Check sheet for the modelled part. Datum: model origin and axes. Units: mm. A direction names the side the tool comes from. Coordinates: 2 decimals unless noted, no trailing zeros. Loops run counter-clockwise (first coordinate to the right, second up) from the corner with the lowest first, then second, coordinate; pieces in that order, holes last. Notation, with made-up numbers: (49, 45) -> (86, 45) arc R11 cw to (86, 50) -> close; hole circle Ø1 at (81, 21). An arc over 180 degrees is marked (long way). Use CSV: the item, a comma, the result in double quotes. Start each with the question number.
1. Set-up check for faces 4 (the face through (69.6, -59.9, 9.7)), 5 (the face through (3, -57.219, 21)), 6 (the face through (68.086, 44.779, 3.346)): record each of +Z, -Z, +X, -X, +Y, -Y from which the full face is reachable in a straight line by a thin tool's end or side.
2. Sectioned sample at A-A, the plane z = 3.75. Record the cut outline in (x, y).
3. Sectioned sample at B-B, the plane y = -40. Record the cut outline in (x, z).
4. Thickness scan on L1, parallel to Y at x = 38, z = 19.75; L2, parallel to X at y = 6.5, z = 21.5; L3, parallel to Y at x = -44, z = 6.5. Record the ranges inside material, lowest first.
5. Release check for a two-part mould opening along Y. For faces 1 (the face through (-66.459, -7, 9)), 2 (the face through (68.941, -7, 3)), 3 (the face through (3, -67.719, 21)) record: pulls with the +Y half, pulls with the -Y half, needs draft (parallel to the pull), parting line crosses it, or undercut.
6. Gauge pin test, flat ends, axial feed: pin 1 (4 mm diameter, centred on x = 52, y = -54, fed in from +Z); pin 2 (5 mm diameter, centred on x = -22.5, z = 12.5, fed in from +Y); pin 3 (8 mm diameter, centred on y = 29, z = 3.5, fed in from -X). Record the tip position at first contact, or that the pin passes through.
7. Sectioned sample at C-C, the plane z = 16. Record the cut outline in (x, y).
8. Sectioned sample at D-D, the plane x = -56. Record the cut outline in (y, z).
Autodesk Inventor part; units mm, degrees
ref_plane "YZ Plane" through (0, 0, 0) normal (1, 0, 0) x (0, 1, 0)
ref_plane "XZ Plane" through (0, 0, 0) normal (0, 1, 0) x (-1, 0, 0)
ref_plane "XY Plane" through (0, 0, 0) normal (0, 0, 1) x (1, 0, 0)
sketch "Sketch1" plane through (0, 0, 0) normal (0, 0, 1) x (1, 0, 0)
  line L0 (-66.4589, 47.2807) -> (70.5411, 47.2807)
  line L1 (70.5411, 47.2807) -> (70.5411, -60.7193)
  line L2 (70.5411, -60.7193) -> (-66.4589, -60.7193)
  line L3 (-66.4589, -60.7193) -> (-66.4589, 47.2807)
  line L4 (68.9411, 45.6807) -> (-64.8589, 45.6807)
  line L5 (-64.8589, 45.6807) -> (-64.8589, -59.1193)
  line L6 (-64.8589, -59.1193) -> (68.9411, -59.1193)
  line L7 (68.9411, -59.1193) -> (68.9411, 45.6807)
  point P0 (0, 0)
  dimension "d0" = 137
  dimension "d1" = 108
  dimension "d2" = 1.6
extrude "Extrusion1" add sketch "Sketch1" along normal blind 19.2 contours L0 L1 L2 L3 | L7 L6 L5 L4
extrude "Extrusion2" cut sketch "Sketch1" along normal blind 6.6 contours L7 L6 L5 L4
sketch "Sketch2" plane through (0, 0, 19.2) normal (0, 0, 1) x (1, 0, 0)
  line L0 (-73.9589, 54.2807) -> (78.0411, 54.2807)
  line L1 (78.0411, 54.2807) -> (78.0411, -67.7193)
  line L2 (78.0411, -67.7193) -> (-73.9589, -67.7193)
  line L3 (-73.9589, -67.7193) -> (-73.9589, 54.2807)
  line L4 (70.5411, 47.2807) -> (-66.4589, 47.2807)
  line L5 (70.5411, -60.7193) -> (70.5411, 47.2807)
  point P0 (0, 0)
  dimension "d7" = 152
  dimension "d8" = 122
  dimension "d9" = 7
  dimension "d10" = 7.5
extrude "Extrusion3" add sketch "Sketch2" along normal blind 3.2
fillet "Fillet1" radius 3 8 edges at (70.5411, 47.2807, 9.6) (-66.4589, 47.2807, 9.6) (70.5411, -60.7193, 9.6) (-66.4589, -60.7193, 9.6) (68.9411, 45.6807, 3.3) (-64.8589, 45.6807, 3.3) (68.9411, -59.1193, 3.3) (-64.8589, -59.1193, 3.3)
fillet "Fillet2" radius 10 4 edges at (-73.9589, 54.2807, 20.8) (-73.9589, -67.7193, 20.8) (78.0411, -67.7193, 20.8) (78.0411, 54.2807, 20.8)
sketch "Sketch3" plane through (0, 0, 22.4) normal (0, 0, 1) x (1, 0, 0)
  arc A0 (78.0411, 44.2807) -> (68.0411, 54.2807) centre (68.0411, 44.2807) ccw
  line L0 (68.0411, 54.2807) -> (-63.9589, 54.2807)
  arc A1 (-63.9589, 54.2807) -> (-73.9589, 44.2807) centre (-63.9589, 44.2807) ccw
  line L1 (-73.9589, 44.2807) -> (-73.9589, -57.7193)
  arc A2 (-73.9589, -57.7193) -> (-63.9589, -67.7193) centre (-63.9589, -57.7193) ccw
  line L2 (-63.9589, -67.7193) -> (68.0411, -67.7193)
  arc A3 (68.0411, -67.7193) -> (78.0411, -57.7193) centre (68.0411, -57.7193) ccw
  line L3 (78.0411, -57.7193) -> (78.0411, 44.2807)
  line L4 (-63.4589, 43.7807) -> (67.5411, 43.7807)
  line L5 (67.5411, 43.7807) -> (67.5411, -57.2193)
  line L6 (67.5411, -57.2193) -> (-63.4589, -57.2193)
  line L7 (-63.4589, -57.2193) -> (-63.4589, 43.7807)
  point P0 (0, 0)
  dimension "d15" = 10.5
extrude "Extrusion4" cut sketch "Sketch3" against normal blind 3 contours L4 L5 L6 L7
equation "\"d9\" = -0.5 * d1 + 0.5 * d8"
equation "\"d10\" = -0.5 * d0 + 0.5 * d7"
properties part number "COTS_Zelmer_108x137mm_HEPA_filter"
Completed:
1,face 4,"-Z, +X, -Y"
1,face 5,"+Z"
1,face 6,"-Z"
2,outline,"(-66.46, -57.72) arc R3 ccw to (-63.46, -60.72) -> (67.54, -60.72) arc R3 ccw to (70.54, -57.72) -> (70.54, 44.28) arc R3 ccw to (67.54, 47.28) -> (-63.46, 47.28) arc R3 ccw to (-66.46, 44.28) -> close; hole (-64.86, -56.12) arc R3 ccw to (-61.86, -59.12) -> (65.94, -59.12) arc R3 ccw to (68.94, -56.12) -> (68.94, 42.68) arc R3 ccw to (65.94, 45.68) -> (-61.86, 45.68) arc R3 ccw to (-64.86, 42.68) -> close"
3,outline,"(-73.96, 19.2) -> (-66.46, 19.2) -> (-66.46, 0) -> (-64.86, 0) -> (-64.86, 6.6) -> (68.94, 6.6) -> (68.94, 0) -> (70.54, 0) -> (70.54, 19.2) -> (78.04, 19.2) -> (78.04, 22.4) -> (67.54, 22.4) -> (67.54, 19.4) -> (-63.46, 19.4) -> (-63.46, 22.4) -> (-73.96, 22.4) -> close"
4,L1,"-67.72 to -57.22, 43.78 to 54.28"
4,L2,"-73.96 to -63.46, 67.54 to 78.04"
4,L3,"-60.72 to -59.12, 45.68 to 47.28"
5,face 1,"needs draft"
5,face 2,"undercut"
5,face 3,"pulls with the -Y half"
6,pin 1,"z = 19.4"
6,pin 2,"y = 47.28"
6,pin 3,"x = -66.46"
7,outline,"(-66.46, -57.72) arc R3 ccw to (-63.46, -60.72) -> (67.54, -60.72) arc R3 ccw to (70.54, -57.72) -> (70.54, 44.28) arc R3 ccw to (67.54, 47.28) -> (-63.46, 47.28) arc R3 ccw to (-66.46, 44.28) -> close"
8,outline,"(-67.72, 19.2) -> (-60.72, 19.2) -> (-60.72, 0) -> (-59.12, 0) -> (-59.12, 6.6) -> (45.68, 6.6) -> (45.68, 0) -> (47.28, 0) -> (47.28, 19.2) -> (54.28, 19.2) -> (54.28, 22.4) -> (43.78, 22.4) -> (43.78, 19.4) -> (-57.22, 19.4) -> (-57.22, 22.4) -> (-67.72, 22.4) -> close"
